Drawing for the job (mm, zero at the part's lowest x, y, z). A direction names the side the tool comes from. Round coordinates to 2 decimals unless told otherwise and drop trailing zeros. Write each loop counter-clockwise with the first axis right and the second up, starting at its lowest first coordinate (ties: lowest second). Pieces come first, ordered by that corner, then holes.
Item 1: Wall check: probe 1 along Y at (x, z) = (93, 28.5); probe 2 along Z at (x, y) = (79, 113.5). Give the ranges that are in metal, low to high.
Item 2: 3-axis set-ups, long thin cutter, end or side, ignore diameter. For the marked faces 5, 6, 7, 8 and 9: which of +Z, -Z, +X, -X, +Y, -Y reach the whole face in a straight line?
Item 3: Band-saw the part on C-C, the plane y = 20. Write the cut outline in (x, z), then the cut area to 3 significant figures.
Item 4: Band-saw the part on D-D, the plane x = 146.5. Write the cut outline in (y, z), then the cut area to 3 significant figures.
Item 5: Band-saw the part on B-B, the plane z = 24. Write the cut outline in (x, y) (3 decimals), then the cut area to 3 significant figures.
Item 6: Mould opens along Y. For the marked faces 1, 2, 3 and 4 say: +Y half, -Y half, draft (parallel to the pull), parting line (faces both ways), or undercut.
Item 7: Band-saw the part on A-A, the plane x = 69. Write the cut outline in (y, z).
Item 8: Drop flat-ended pins along their axis: pin 1 Ø4 at (y, z) = (61, 33) entering from +X; pin 2 Ø14 at (y, z) = (117, 12.5) entering from -X; pin 3 Ø6.5 at (y, z) = (116, 29) entering from +X; pin 4 Ø4 at (y, z) = (114, 45) entering from -X. Give the stop position or say it passes through.
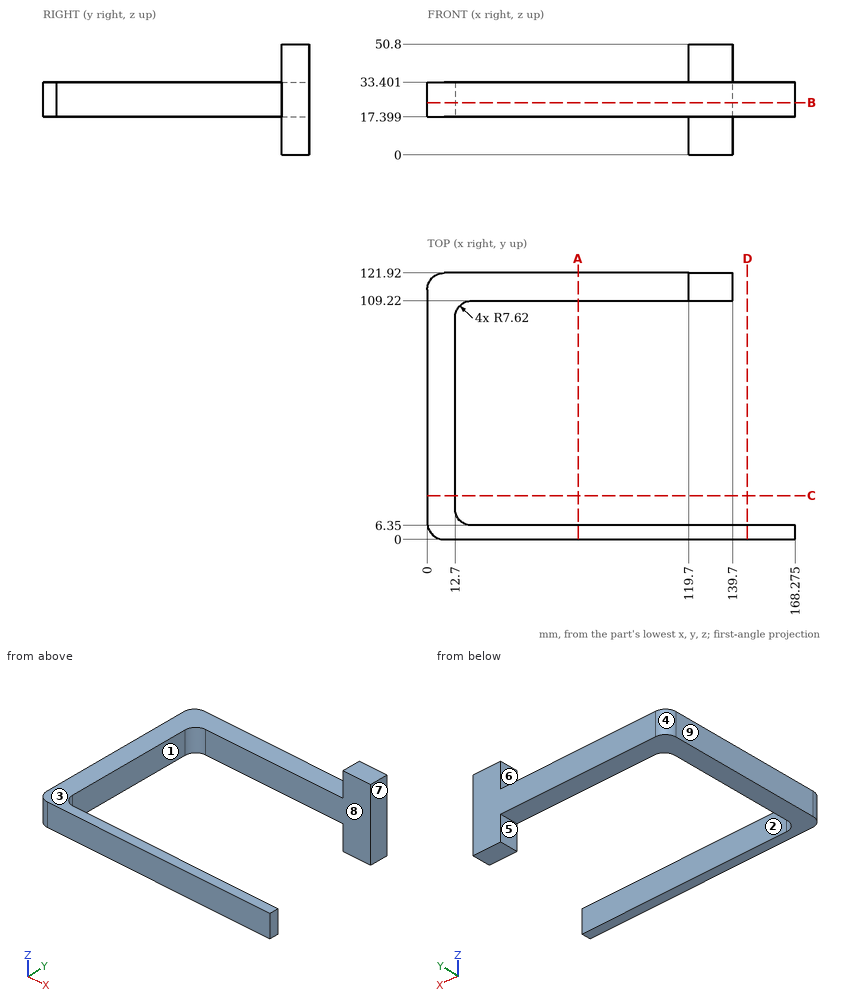
Results:
1. probe 1: y = 0 to 6.35, 109.22 to 121.92
1. probe 2: z = 17.4 to 33.4
2. face 5: -Z, -X, +Y, -Y
2. face 6: +Z, -X, +Y, -Y
2. face 7: +Z, -Z, +X, +Y
2. face 8: +Z, -Z, +X
2. face 9: +Z, -Z, -X, +Y, -Y
3. outline: (0, 17.4) - (12.7, 17.4) - (12.7, 33.4) - (0, 33.4) - close
3. area: 203 mm2
4. outline: (0, 17.4) - (6.35, 17.4) - (6.35, 33.4) - (0, 33.4) - close
4. area: 102 mm2
5. outline: (0, 7.62) arc R7.62 ccw to (7.62, 0) - (168.275, 0) - (168.275, 6.35) - (20.32, 6.35) arc R7.62 cw to (12.7, 13.97) - (12.7, 101.6) arc R7.62 cw to (20.32, 109.22) - (139.7, 109.22) - (139.7, 121.92) - (7.62, 121.92) arc R7.62 ccw to (0, 114.3) - close
5. area: 4,150 mm2
6. face 1: undercut
6. face 2: undercut
6. face 3: draft
6. face 4: +Y half
7. outline: (0, 17.4) - (6.35, 17.4) - (6.35, 33.4) - (0, 33.4) - close; (109.22, 17.4) - (121.92, 17.4) - (121.92, 33.4) - (109.22, 33.4) - close
8. pin 1: stops at x = 12.7
8. pin 2: stops at x = 0
8. pin 3: stops at x = 139.7
8. pin 4: stops at x = 119.7
